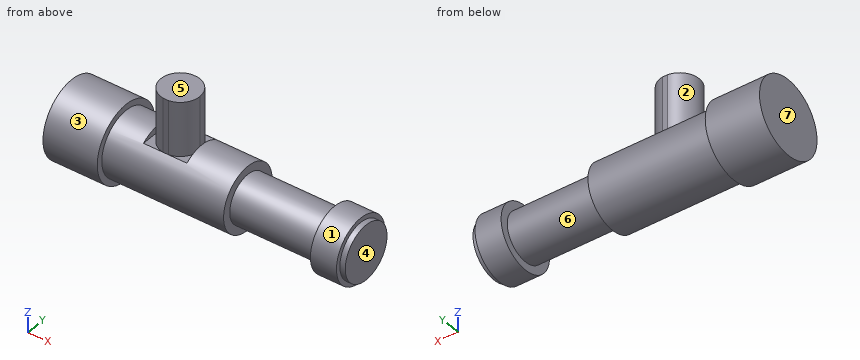
```python
from build123d import *

# Parameters (mm, degrees)
F2_W     = 20
F2_H     = 3
F3_DEPTH = 10.1
F5_DEPTH = 25


with BuildPart() as f1:
    # F0 (on Front) → F1 (revolve)
    with BuildSketch(Plane.XZ):
        Polygon((-81.1, 0), (54.5, 0), (54.5, 12.7), (52, 12.7), (52, 14.75), (40, 14.75), (40, 11), (0, 11), (0, 14.75), (-56.1, 14.75), (-56.1, 17.5), (-81.1, 17.5), align=None)
    revolve(axis=Axis((-19.562621, 0, 0), (-1, 0, 0)))

    # F2 (on Front) → F3 (cut, symmetric)
    with BuildSketch(Plane.XZ):
        with Locations((-31.3, 13.25)):
            Rectangle(F2_W, F2_H)
    extrude(amount=F3_DEPTH, both=True, mode=Mode.SUBTRACT)

    # F4 (on face) → F5 (join)
    with BuildSketch(Plane.XY.offset(11.75)):
        with BuildLine():
            ThreePointArc((-29.875255, -8.916277), (-24.316833, -5.91512), (-22.1, 0))
            ThreePointArc((-22.1, 0), (-24.316833, 5.91512), (-29.875255, 8.916277))
            Line((-29.875255, 8.916277), (-32.324745, 8.916277))
            ThreePointArc((-32.324745, 8.916277), (-40.1, 0), (-32.324745, -8.916277))
            Line((-32.324745, -8.916277), (-29.875255, -8.916277))
        make_face()
    extrude(amount=F5_DEPTH)


solid = f1.part
```
Read the model definition and answer for the solid it produces. Units are mm, in the model's axes. Face numbers are marked on the shaded views. A direction names the side the tool comes from. Give positions to 0.01 mm unless a question says otherwise; leave off trailing zeros. Loops run counter-clockwise (first coordinate to the right, second up) from the corner with the lowest first, then second, coordinate; pieces in that order, holes last.
Item 1: The part is cut by section A-A (z = 0). Write down the section's boundary in (x, y), and give its area (3 significant figures).
Item 2: The mould has two halves that part along X. Classify the marked faces 4, 5, 6 and 7: released by +X, released by -X, zero draft, split by the parting line, or undercut.
Item 3: Find the intervals of material crossed by line 1 along X through (y, z) = (3, 13); line 2 along X through (y, z) = (-11, 6); line 3 along X through (y, z) = (13, -8), in increasing order.
Item 4: Each of these flat-tipped pins is pushed along its axis until it touches: pin 1 Ø0.7 at (x, z) = (-31.5, 21.5) entering from +Y; pin 2 Ø2 at (x, z) = (-5.5, -9) entering from -Y; pin 3 Ø1 at (y, z) = (-12, 9) entering from +X. Where does it stop, or does it pass through?
Item 5: For the marked faces 1, 2 and 3, determine the directions among +Z, -Z, +X, -X, +Y, -Y from which every point of the face is accessible in a straight line to the end or side of a thin tool.
Item 6: The part is cut by section D-D (z = 23). Write down the section's boundary in (x, y).
Item 7: The part is cut by section B-B (y = -7). Write down the section's boundary in (x, z), and give its area (3 significant figures).
Item 8: The part is cut by section C-C (x = -36). Write down the section's boundary in (y, z).
Taken from the geometry:
1. outline: (-81.1, -17.5) - (-56.1, -17.5) - (-56.1, -14.75) - (0, -14.75) - (0, -11) - (40, -11) - (40, -14.75) - (52, -14.75) - (52, -12.7) - (54.5, -12.7) - (54.5, 12.7) - (52, 12.7) - (52, 14.75) - (40, 14.75) - (40, 11) - (0, 11) - (0, 14.75) - (-56.1, 14.75) - (-56.1, 17.5) - (-81.1, 17.5) - close
1. area: 3,830 mm2
2. face 4: released by +X
2. face 5: zero draft
2. face 6: undercut
2. face 7: released by -X
3. line 1: x = -81.1 to -41.3, -39.59 to -22.61, -21.3 to 0, 40 to 52
3. line 2: x = -81.1 to 0, 40 to 54.5
3. line 3: x = -81.1 to -56.1
4. pin 1: stops at y = 8.92
4. pin 2: stops at y = -12.39
4. pin 3: stops at x = 52
5. face 1: +X
5. face 2: +Z
5. face 3: -X
6. outline: (-32.32, -8.92) - (-29.88, -8.92) arc R9 ccw to (-29.88, 8.92) - (-32.32, 8.92) arc R9 ccw to start
7. outline: (-81.1, -16.04) - (-56.1, -16.04) - (-56.1, -12.98) - (0, -12.98) - (0, -8.49) - (40, -8.49) - (40, -12.98) - (52, -12.98) - (52, -10.6) - (54.5, -10.6) - (54.5, 10.6) - (52, 10.6) - (52, 12.98) - (40, 12.98) - (40, 8.49) - (0, 8.49) - (0, 12.98) - (-21.3, 12.98) - (-21.3, 11.75) - (-25.44, 11.75) - (-25.44, 36.75) - (-36.76, 36.75) - (-36.76, 11.75) - (-41.3, 11.75) - (-41.3, 12.98) - (-56.1, 12.98) - (-56.1, 16.04) - (-81.1, 16.04) - close
7. area: 3,560 mm2
8. outline: (-8.92, 11.75) arc R14.75 ccw (long way) to (8.92, 11.75) - (7.55, 11.75) - (7.55, 36.75) - (-7.55, 36.75) - (-7.55, 11.75) - close
